The model under review builds one solid part; all positions refer to its coordinate system, in mm. Face numbers are marked on the shaded views. A direction names the side the tool comes from. Coordinates: 2 decimals unless noted, no trailing zeros. Order: outer loops, then holes, each group sorted by start corner. A loop starts at its lowest first (then second) coordinate and runs counter-clockwise, first axis right, second up. Notation, with made-up numbers: (70.5, 1) -> (126.5, 1) arc R15 cw to (126.5, 7) -> close; hole circle Ø2 at (64, 24). An arc over 180 degrees is marked (long way). Use one line per item in the form item = value. Start each with the question number.
(1) Take a section at A-A (z = 3.5). State the section outline as (x, y) points.
(2) Wall thickness on line 1 along Y through (x, z) = (1, 4.25); line 2 along Z through (x, y) = (6.75, 1.5); line 3 along X through (y, z) = (8.5, 3): over which ranges is each line inside the solid? List them lowest first.
(3) Mouldability with a two-part tool opening along X and no side actions: class the marked faces 1, 2 and 3 as +X half, -X half, draft (parallel to the pull), parting line (faces both ways), or undercut.
(4) For the marked faces 4, 5 and 6, list the 3-axis set-ups (+Z, -Z, +X, -X, +Y, -Y) from which the entire face can be reached by the end or side of a thin tool; tool diameter is ignored.
(5) Insertion check: pin 1 Ø1.8 at (x, z) = (5, 3.5) entering from +Y; pin 2 Ø3 at (y, z) = (7.5, 4) entering from +X; pin 3 Ø5 at (x, y) = (3, 4.5) entering from +Z. Each pin has a flat end and moves straight along its axis. Give the tip position at first contact, or say it passes through.
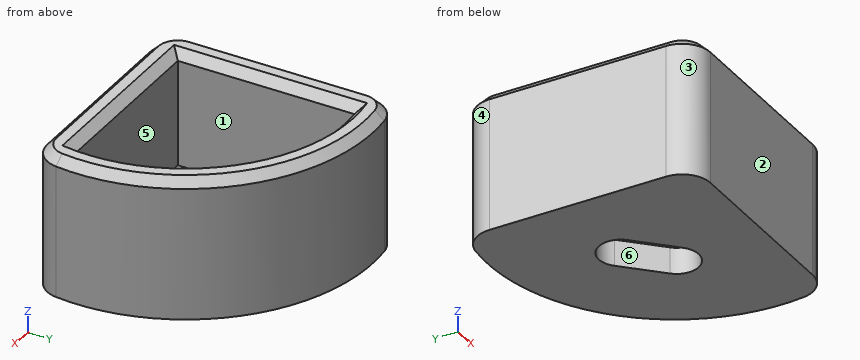
```python
from build123d import *

# Parameters (mm, degrees)
EXTRUDE_1_DEPTH     = 8
CUT_EXTRUDE_1_DEPTH = 6.5
CUT_EXTRUDE_2_DEPTH = 18.728535031
FILLET_1_R          = 1.6
CHAMFER_2_SIZE      = 0.5


with BuildPart() as part:
    # 草图1 → 凸台-拉伸1 (new body)
    with BuildSketch(Plane.XY):
        with BuildLine():
            Line((-1.6, -1.6), (11.323037582, -1.6))
            ThreePointArc((11.323037582, -1.6), (8.558327944, 8.558327944), (-1.6, 11.323037582))
            Line((-1.6, 11.323037582), (-1.6, -1.6))
        make_face()
    extrude(amount=EXTRUDE_1_DEPTH)

    # 草图2 → 切除-拉伸1 (cut)
    with BuildSketch(Plane.XY.offset(8)):
        with BuildLine():
            Line((0, 0), (10, 0))
            ThreePointArc((10, 0), (7.426957094, 7.426957094), (0, 10))
            Line((0, 10), (0, 0))
        make_face()
    extrude(amount=-CUT_EXTRUDE_1_DEPTH, mode=Mode.SUBTRACT)

    # 草图5 → 切除-拉伸2 (cut, through all)
    with BuildSketch(Plane.XY.offset(1.5)):
        with BuildLine():
            Line((2.616116524, 4.616116524), (4.616116524, 2.616116524))
            ThreePointArc((4.616116524, 2.616116524), (6.383883476, 2.616116524), (6.383883476, 4.383883476))
            Line((6.383883476, 4.383883476), (4.383883476, 6.383883476))
            ThreePointArc((4.383883476, 6.383883476), (2.616116524, 6.383883476), (2.616116524, 4.616116524))
        make_face()
    extrude(amount=-CUT_EXTRUDE_2_DEPTH, mode=Mode.SUBTRACT)

    # 圆角1
    fillet_1_edges = [part.edges().sort_by_distance(p)[0] for p in [
        (-1.6, 11.323037582, 4),
        (11.323037582, -1.6, 4),
        (-1.6, -1.6, 4),
    ]]
    fillet(fillet_1_edges, radius=FILLET_1_R)

    # 倒角2
    chamfer_2_edges = [part.edges().sort_by_distance(p)[0] for p in [
        (0, 5, 8),
        (5, 0, 8),
        (7.426957094, 7.426957094, 8),
        (-1.6, 5, 8),
        (8.558327944, 8.558327944, 8),
        (5, -1.6, 8),
        (11.062458629, -1.19632005, 8),
        (-1.13137085, -1.13137085, 8),
        (-1.19632005, 11.062458629, 8),
    ]]
    chamfer(chamfer_2_edges, length=CHAMFER_2_SIZE)


solid = part.part
```
Findings:
q1.outline = (-1.6, 0) arc R1.6 ccw to (0, -1.6) -> (10, -1.6) arc R1.6 ccw to (11.59, -0.19) arc R10.6 ccw to (-0.19, 11.59) arc R1.6 ccw to (-1.6, 10) -> close; hole (0, 0) -> (10, 0) arc R9 ccw to (0, 10) -> close
q2.line_1 = -1.6 to 0, 10.06 to 11.66
q2.line_2 = 0 to 1.5
q2.line_3 = -1.6 to 0, 6.13 to 8.62
q3.face_1 = undercut
q3.face_2 = draft
q3.face_3 = -X half
q4.face_4 = +Z, -Z, -X, +Y
q4.face_5 = +Z
q4.face_6 = +Z, -Z
q5.pin_1 = 11.22
q5.pin_2 = 10.44
q5.pin_3 = 1.5
